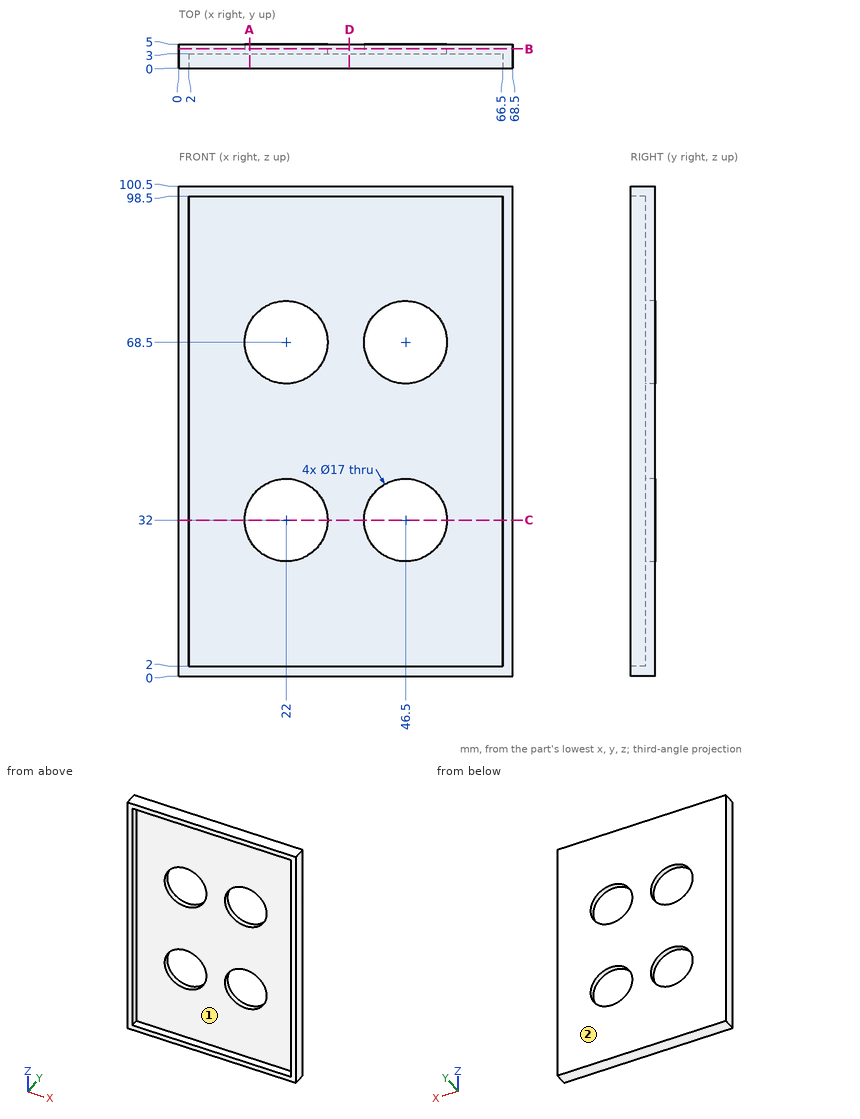
Drawing for the job (mm, zero at the part's lowest x, y, z). Round coordinates to 2 decimals unless told otherwise and drop trailing zeros. Loops run counter-clockwise (first coordinate to the right, second up) from the corner with the lowest first, then second, coordinate; pieces in that order, holes last. Notation, with made-up numbers: (54, 43) -> (90, 43) arc R21 cw to (90, 64) -> close; hole circle Ø6 at (37, 24.5). An arc over 180 degrees is marked (long way). Answer as CSV lines item,"result". Start each with the question number.
1) Pin check, flat tips, straight feed: P1, Ø10, axis at x = 22, z = 68.5, coming from the -Y side; P2, Ø22, axis at x = 22, z = 32, coming from the -Y side; P3, Ø2.5, axis at x = 42.5, y = 1.5, coming from the -Z side. Stop position of each tip, or through.
2) Mould opens along X. For the marked faces 1 and 2 say: +X half, -X half, draft (parallel to the pull), parting line (faces both ways), or undercut.
3) Slice it at A-A (x = 14.5). List the corners of the cut face in (y, z), plus the area to 3 significant figures.
4) Slice it at D-D (x = 35). List the corners of the cut face in (y, z), plus the area to 3 significant figures.
5) Probe line 1 along X through (y, z) = (4.3, 32); line 2 along Z through (x, y) = (22, 4.6); line 3 along Z through (x, y) = (40, 1.4). List the from-to ranges inside material, lowest first.
6) Slice it at C-C (z = 32). List the corners of the cut face in (x, y), plus the area to 3 significant figures.
7) Slice it at B-B (y = 4). List the corners of the cut face in (x, z), plus the area to 3 significant figures.
Filled in:
1,P1,"passes through"
1,P2,"stops at y = 3"
1,P3,"stops at z = 0"
2,face 1,"undercut"
2,face 2,"draft"
3,outline,"(0, 0) -> (5, 0) -> (5, 28) -> (3, 28) -> (3, 2) -> (0, 2) -> close; (0, 98.5) -> (3, 98.5) -> (3, 72.5) -> (5, 72.5) -> (5, 100.5) -> (0, 100.5) -> close; (3, 36) -> (5, 36) -> (5, 64.5) -> (3, 64.5) -> close"
3,area,"181 mm2"
4,outline,"(0, 0) -> (5, 0) -> (5, 100.5) -> (0, 100.5) -> (0, 98.5) -> (3, 98.5) -> (3, 2) -> (0, 2) -> close"
4,area,"213 mm2"
5,line 1,"x = 0 to 13.5, 30.5 to 38, 55 to 68.5"
5,line 2,"z = 0 to 23.5, 40.5 to 60, 77 to 100.5"
5,line 3,"z = 0 to 2, 98.5 to 100.5"
6,outline,"(0, 0) -> (2, 0) -> (2, 3) -> (13.5, 3) -> (13.5, 5) -> (0, 5) -> close; (30.5, 3) -> (38, 3) -> (38, 5) -> (30.5, 5) -> close; (55, 3) -> (66.5, 3) -> (66.5, 0) -> (68.5, 0) -> (68.5, 5) -> (55, 5) -> close"
6,area,"81.0 mm2"
7,outline,"(0, 0) -> (68.5, 0) -> (68.5, 100.5) -> (0, 100.5) -> close; hole circle Ø17 at (22, 32); hole circle Ø17 at (22, 68.5); hole circle Ø17 at (46.5, 32); hole circle Ø17 at (46.5, 68.5)"
7,area,"5,980 mm2"
